Here's how the part is built. I have some questions about the finished solid (model axes, mm). A direction names the side the tool comes from. Give positions to 0.01 mm unless a question says otherwise; leave off trailing zeros. Loops run counter-clockwise (first coordinate to the right, second up) from the corner with the lowest first, then second, coordinate; pieces in that order, holes last.
Q1. Suppose I cut it at A-A (y = 1.25). List the corners of the cut face in (x, z) for me (3 decimals).
Q2. I need wall thicknesses on probe 1 along X at (y, z) = (-1.75, 25); probe 2 along Z at (x, y) = (5, 3) (3 decimals); probe 3 along X at (y, z) = (2, -33). Which ranges of each line are inside material? Lowest first, please.
Q3. Thinking about a two-plate mould opening in Z: for faces 1 (the face through (-14.7, -0.2, 0.5)), 2 (the face through (1, 0, 0)), 3 (the face through (0, 1, 36.925)), which applies, pulls with the +Z half, pulls with the -Z half, needs draft (parallel to the pull), parting line crosses it, or undercut?
Q4. Suppose I cut it at C-C (z = 6). List the corners of the cut face in (x, y) for me.
Q5. For faces 4 (the face through (-13.2, 2, 0)), 5 (the face through (15.01, 2.23, -0.11)), 6 (the face through (14, 2, 8.075)), 7 (the face through (-9.074, -1.521, 26.356)), 8 (the face through (1.5, 2, -36)), which set-ups out of +Z, -Z, +X, -X, +Y, -Y let a thin tool reach every point of the face, with its end or its side?
Q6. I'm going to push flat-ended pins straight in: P1, Ø0.5, axis at x = 15, y = 2, coming from the -Z side; P2, Ø14, axis at x = 0.5, z = -6, coming from the +Y side; P3, Ø0.5, axis at x = -15, y = 3, coming from the +Z side. Where does each tip first touch, or does it pass through?
Q7. Suppose I cut it at D-D (x = -4). List the corners of the cut face in (y, z) for me (3 decimals), and give its area (3 significant figures).
Q8. Suppose I cut it at B-B (x = 0). List the corners of the cut face in (y, z) for me (3 decimals).
```python
from build123d import *

# Parameters (mm, degrees)
SKETCH1_W               = 29.4
SKETCH1_H               = 73.85
SKETCH1_W_2             = 26.4
SKETCH1_H_2             = 70.85
SKETCH1_W_3             = 25.4
SKETCH1_H_3             = 69.85
BOSS_EXTRUDE1_DEPTH     = 3
SKETCH1_3_W             = 29.4
SKETCH1_3_H             = 73.85
SKETCH1_3_W_2           = 26.4
SKETCH1_3_H_2           = 70.85
BOSS_EXTRUDE2_DEPTH     = 4.4
CUT_EXTRUDE1_DEPTH      = 40.986317973
CUT_EXTRUDE1_DEPTH_BACK = 40.986317973
SKETCH2_R               = 1.5
SKETCH3_W               = 3
SKETCH3_H               = 4.5
CUT_EXTRUDE2_DEPTH      = 1.5
SKETCH4_W               = 12
SKETCH4_H               = 4.4
CUT_EXTRUDE3_DEPTH      = 1.5
SKETCH5_W               = 15
SKETCH5_H               = 4.4
BOSS_EXTRUDE3_DEPTH     = 1
CHAMFER1_SIZE           = 1
CHAMFER1_SIZE_2         = 7
CHAMFER2_SIZE           = 1
CHAMFER2_SIZE_2         = 7


with BuildPart() as part:
    # Sketch1 → Boss-Extrude1 (new body)
    # profile 1 of 3: a face of its own
    with BuildSketch(Plane(origin=(0, 0, 0), x_dir=(1, 0, 0), z_dir=(0, 1, 0))):
        Rectangle(SKETCH1_W, SKETCH1_H)
        Rectangle(SKETCH1_W_2, SKETCH1_H_2, mode=Mode.SUBTRACT)
    # profile 2 of 3: a face of its own
    with BuildSketch(Plane(origin=(0, 0, 0), x_dir=(1, 0, 0), z_dir=(0, 1, 0))):
        Rectangle(SKETCH1_W_2, SKETCH1_H_2)
        Rectangle(SKETCH1_W_3, SKETCH1_H_3, mode=Mode.SUBTRACT)
    # profile 3 of 3: a face of its own
    with BuildSketch(Plane(origin=(0, 0, 0), x_dir=(1, 0, 0), z_dir=(0, 1, 0))):
        Rectangle(SKETCH1_W_3, SKETCH1_H_3)
    extrude(amount=-BOSS_EXTRUDE1_DEPTH)

    # Sketch1<3> → Boss-Extrude2 (add)
    with BuildSketch(Plane(origin=(0, 0, 0), x_dir=(1, 0, 0), z_dir=(0, 1, 0))):
        Rectangle(SKETCH1_3_W, SKETCH1_3_H)
        Rectangle(SKETCH1_3_W_2, SKETCH1_3_H_2, mode=Mode.SUBTRACT)
    extrude(amount=BOSS_EXTRUDE2_DEPTH)

    # Sketch2 → Cut-Extrude1 (cut, two sides: drawn at the far end of the back side and taken through both)
    with BuildSketch(Plane(origin=(0, 0, 0), x_dir=(1, 0, 0), z_dir=(0, 1, 0)).offset(-CUT_EXTRUDE1_DEPTH_BACK)):
        with BuildLine():
            ThreePointArc((11.025, 32.225), (9.525, 33.725), (8.025, 32.225))
            Line((8.025, 32.225), (9.525, 32.225))
            Line((9.525, 32.225), (9.525, 30.725))
            ThreePointArc((9.525, 30.725), (10.585660172, 31.164339828), (11.025, 32.225))
        make_face()
        with BuildLine():
            Line((9.525, 32.225), (8.025, 32.225))
            ThreePointArc((8.025, 32.225), (8.464339828, 31.164339828), (9.525, 30.725))
            Line((9.525, 30.725), (9.525, 32.225))
        make_face()
        with Locations(Location((-9.525, 32.225, 0), (0, 0, 270))):
            Circle(SKETCH2_R)
        with Locations(Location((-9.525, -24.925, 0), (0, 0, 270))):
            Circle(SKETCH2_R)
        with Locations(Location((9.525, -24.925, 0), (0, 0, 270))):
            Circle(SKETCH2_R)
    extrude(amount=CUT_EXTRUDE1_DEPTH + CUT_EXTRUDE1_DEPTH_BACK, mode=Mode.SUBTRACT)

    # Sketch3 → Cut-Extrude2 (cut)
    with BuildSketch(Plane(origin=(0, 0, -36.925), x_dir=(-1, 0, 0), z_dir=(0, 0, -1))):
        with Locations((0, 2.15)):
            Rectangle(SKETCH3_W, SKETCH3_H)
    extrude(amount=-CUT_EXTRUDE2_DEPTH, mode=Mode.SUBTRACT)

    # Sketch4 → Cut-Extrude3 (cut)
    with BuildSketch(Plane.ZY.offset(-13.2)):
        with Locations((14.075, 2.2)):
            Rectangle(SKETCH4_W, SKETCH4_H)
    extrude(amount=-CUT_EXTRUDE3_DEPTH, mode=Mode.SUBTRACT)

    # Sketch5 → Boss-Extrude3 (add)
    with BuildSketch(Plane.ZY.offset(14.7)):
        with Locations((0, 2.2)):
            Rectangle(SKETCH5_W, SKETCH5_H)
    boss_extrude3 = extrude(amount=BOSS_EXTRUDE3_DEPTH)

    # Chamfer1
    # the kernel refuses this chamfer: 7, 1 mm, written as the material it takes off along each edge
    with BuildSketch(Plane(origin=(-15.7, 4.4, -25.693233978), x_dir=(0.9662442572155542, 0.2576277069687226, 0), z_dir=(0, 0, 1))) as chamfer1_piece_1:
        Polygon((CHAMFER1_SIZE * 0.966244257216, -CHAMFER1_SIZE * 0.257627706969), (-CHAMFER1_SIZE_2 * 0.257627706969, -CHAMFER1_SIZE_2 * 0.966244257216), (0, 0), align=None)
    extrude(amount=51.386467957, mode=Mode.SUBTRACT)

    # Mirror1: Boss-Extrude3 across plane
    add(boss_extrude3.mirror(Plane(origin=(0, 0, 0), x_dir=(0, 0, 1), z_dir=(1, 0, 0))))

    # Chamfer2
    # the kernel refuses this chamfer: 7, 1 mm, written as the material it takes off along each edge
    with BuildSketch(Plane(origin=(15.7, 4.4, -25.693233978), x_dir=(-0.9662442572155542, 0.2576277069687226, 0), z_dir=(0, 0, 1))) as chamfer2_piece_1:
        Polygon((CHAMFER2_SIZE * 0.966244257216, CHAMFER2_SIZE * 0.257627706969), (-CHAMFER2_SIZE_2 * 0.257627706969, CHAMFER2_SIZE_2 * 0.966244257216), (0, 0), align=None)
    extrude(amount=51.386467957, mode=Mode.SUBTRACT)


solid = part.part
```
Solutions:
1. outline: (-15.15, -7.5) - (-14.7, -7.5) - (-14.7, -36.925) - (-1.5, -36.925) - (-1.5, -35.425) - (-13.2, -35.425) - (-13.2, 35.425) - (13.2, 35.425) - (13.2, 20.075) - (14.7, 20.075) - (14.7, 36.925) - (-14.7, 36.925) - (-14.7, 7.5) - (-15.15, 7.5) - close; (1.5, -36.925) - (14.7, -36.925) - (14.7, -7.5) - (15.15, -7.5) - (15.15, 7.5) - (14.7, 7.5) - (14.7, 8.075) - (13.2, 8.075) - (13.2, -35.425) - (1.5, -35.425) - close
2. probe 1: x = -14.7 to -11.02, -8.03 to 8.03, 11.02 to 14.7
2. probe 2: z = -36.925 to -35.425, 35.425 to 36.925
2. probe 3: x = -14.7 to -13.2, 13.2 to 14.7
3. face 1: needs draft
3. face 2: undercut
3. face 3: pulls with the +Z half
4. outline: (-15.33, 0) - (-14.7, 0) - (-14.7, -3) - (14.7, -3) - (14.7, 0) - (15.33, 0) - (14.7, 4.4) - (13.2, 4.4) - (13.2, 0) - (-13.2, 0) - (-13.2, 4.4) - (-14.7, 4.4) - close
5. face 4: +Y
5. face 5: +Z, -Z, +X, +Y
5. face 6: +X, +Y
5. face 7: +Y, -Y
5. face 8: -Z, +Y
6. P1: stops at z = -7.5
6. P2: stops at y = 0
6. P3: stops at z = 7.5
7. outline: (-3, -36.925) - (4.4, -36.925) - (4.4, -35.425) - (0, -35.425) - (0, 35.425) - (4.4, 35.425) - (4.4, 36.925) - (-3, 36.925) - close
7. area: 235 mm2
8. outline: (-3, -36.925) - (-0.1, -36.925) - (-0.1, -35.425) - (0, -35.425) - (0, 35.425) - (4.4, 35.425) - (4.4, 36.925) - (-3, 36.925) - close
